Check sheet for the modelled part. Datum: model origin and axes. Units: mm. Face numbers are marked on the shaded views. A direction names the side the tool comes from. Round coordinates to 2 decimals unless told otherwise and drop trailing zeros. Write each loop counter-clockwise with the first axis right and the second up, starting at its lowest first coordinate (ties: lowest second). Pieces come first, ordered by that corner, then holes. Notation, with made-up numbers: (-2, 14.5) -> (34, 14.5) arc R30 cw to (34, 53.5) -> close; hole circle Ø9 at (40.25, 7). An arc over 180 degrees is marked (long way). Write item = value, one per line.
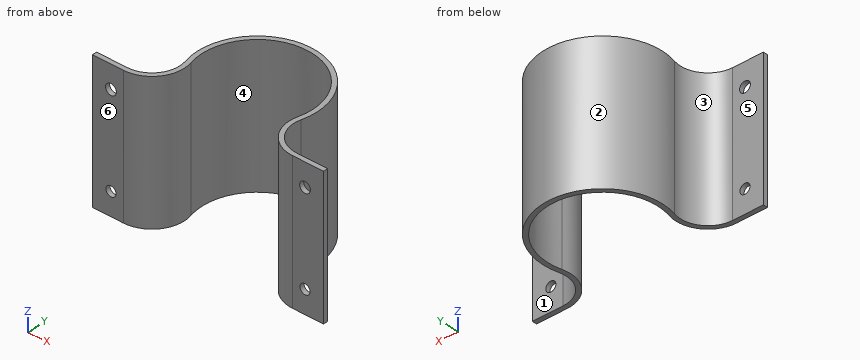
from build123d import *

# Parameters (mm, degrees)
BOSS_EXTRUDE1_DEPTH = 30
SKETCH2_R           = 1.089483659
SKETCH2_R_2         = 1.173994866
CUT_EXTRUDE1_DEPTH  = 15


with BuildPart() as part:
    # Sketch1 → Boss-Extrude1 (new body)
    with BuildSketch(Plane.XY):
        with BuildLine():
            Line((-25, -12), (-18.33030278, -12))
            ThreePointArc((-18.33030278, -12), (-12.76726688, -9.248838851), (-11.577033335, -3.157894737))
            ThreePointArc((-11.577033335, -3.157894737), (0, 12), (11.577033335, -3.157894737))
            ThreePointArc((11.577033335, -3.157894737), (12.76726688, -9.248838851), (18.33030278, -12))
            Line((18.33030278, -12), (25, -12))
            Line((25, -12), (25, -11))
            Line((25, -11), (18.33030278, -11))
            ThreePointArc((18.33030278, -11), (13.561986294, -8.641861872), (12.541786113, -3.421052632))
            ThreePointArc((12.541786113, -3.421052632), (0, 13), (-12.541786113, -3.421052632))
            ThreePointArc((-12.541786113, -3.421052632), (-13.561986294, -8.641861872), (-18.33030278, -11))
            Line((-18.33030278, -11), (-25, -11))
            Line((-25, -11), (-25, -12))
        make_face()
    extrude(amount=BOSS_EXTRUDE1_DEPTH)

    # Sketch2 → Cut-Extrude1 (cut)
    with BuildSketch(Plane(origin=(0, -11, 0), x_dir=(1, 0, 0), z_dir=(0, 1, 0))):
        with Locations((21, -5)):
            Circle(SKETCH2_R)
        with Locations((21, -25)):
            Circle(SKETCH2_R_2)
    cut_extrude1 = extrude(amount=-CUT_EXTRUDE1_DEPTH, mode=Mode.SUBTRACT)

    # Mirror1: Cut-Extrude1 across plane
    add(cut_extrude1.mirror(Plane(origin=(0, 0, 0), x_dir=(0, 0, 1), z_dir=(1, 0, 0))), mode=Mode.SUBTRACT)


solid = part.part
(1) Sectioned sample at D-D on y = 6.75. Enter the section's corners in (x, z).
Worked answers:
outline = (-11.11, 0) -> (-9.92, 0) -> (-9.92, 30) -> (-11.11, 30) -> close; (9.92, 0) -> (11.11, 0) -> (11.11, 30) -> (9.92, 30) -> close
(2) Release check for a two-part mould opening along Y. For the marked faces 3, 4, 5 and 6 record: pulls with the +Y half, pulls with the -Y half, needs draft (parallel to the pull), parting line crosses it, or undercut.
Worked answers:
face_3 = undercut
face_4 = undercut
face_5 = pulls with the +Y half
face_6 = pulls with the -Y half
(3) Sectioned sample at B-B on y = 0. Enter the section's corners in (x, z), then the cut area to 3 significant figures.
Worked answers:
outline = (-13, 0) -> (-12, 0) -> (-12, 30) -> (-13, 30) -> close; (12, 0) -> (13, 0) -> (13, 30) -> (12, 30) -> close
area = 60.0 mm²
(4) Go/stop test with flat-tipped pins: P1, Ø2.5, axis at x = -21, z = 5, coming from the +Y side; P2, Ø4, axis at y = 5.5, z = 14.5, coming from the +X side; P3, Ø4, axis at x = 11.5, z = 16.5, coming from the +Y side. Record where each tip stops, or that it passes through.
Worked answers:
P1 = -11
P2 = 12.52
P3 = 8.87
(5) Access from +Z, -Z, +X, -X, +Y, -Y to the whole of each face (thin tool, end or side, straight path). Record for the marked faces 1 and 2.
Worked answers:
face_1 = +Z, -Z, +X, +Y
face_2 = +Z, -Z
(6) Sectioned sample at A-A on x = 21. Enter the section's corners in (y, z), then the cut area to 3 significant figures.
Worked answers:
outline = (-12, 0) -> (-11, 0) -> (-11, 3.91) -> (-12, 3.91) -> close; (-12, 6.09) -> (-11, 6.09) -> (-11, 23.83) -> (-12, 23.83) -> close; (-12, 26.17) -> (-11, 26.17) -> (-11, 30) -> (-12, 30) -> close
area = 25.5 mm²
(7) Material ranges on L1, parallel to Z at x = 21, y = -11.7; L2, parallel to X at y = 0, z = 17.5; L3, parallel to X at y = -11.3, z = 25, recorded low to high. Write a range as [from, to].
Worked answers:
L1 = [0, 3.91], [6.09, 23.83], [26.17, 30]
L2 = [-13, -12], [12, 13]
L3 = [-25, -22.17], [-19.83, -15.28], [15.28, 19.83], [22.17, 25]
(8) Sectioned sample at C-C on z = 9.5. Enter the section's corners in (x, y).
Worked answers:
outline = (-25, -12) -> (-18.33, -12) arc R7 ccw to (-11.58, -3.16) arc R12 cw (long way) to (11.58, -3.16) arc R7 ccw to (18.33, -12) -> (25, -12) -> (25, -11) -> (18.33, -11) arc R6 cw to (12.54, -3.42) arc R13 ccw (long way) to (-12.54, -3.42) arc R6 cw to (-18.33, -11) -> (-25, -11) -> close
